For this review, take the finished solid that the model builds, in its own axes (mm). Give positions to 0.01 mm unless a question says otherwise; leave off trailing zeros. Order: outer loops, then holes, each group sorted by start corner. A loop starts at its lowest first (then second) coordinate and runs counter-clockwise, first axis right, second up. Notation, with made-up numbers: M 1,11.25 L 11,11.25 A23 ccw 11,50.25 Z; hole C 70,-22 d9. An arc over 180 degrees is marked long. Answer as CSV lines item,"result". Start each with the question number.
1. Clearance check with flat-ended pins moving along their axes: P1, Ø1.5, axis at y = -1, z = -24, coming from the -X side; P2, Ø1.5, axis at y = -1.5, z = -10, coming from the +X side. State where each tip first meets the part, or that it passes through.
2. For line 1 along X through (y, z) = (-0.2, -17); line 2 along Z through (x, y) = (39.5, -1.1); line 3 along Z through (x, y) = (-22.5, -0.4), list the stretches that pass through material, from the lowest coordinate up.
3. We need section B-B, the plane z = -11. Give the boundary of the cut face in (x, y).
4. We need section C-C, the plane y = -2.55. State how many separate pieces and enclosed holes the cut face has, and give its area (3 significant figures).
5. We need section D-D, the plane z = -28. Give the boundary of the cut face in (x, y).
6. We need section A-A, the plane x = -39. Give the boundary of the cut face in (y, z).
from build123d import *

# Parameters (mm, degrees)
SKETCH1_W          = 2.9
SKETCH1_H          = 5
SKETCH1_W_2        = 6
BASE_FLANGE1_DEPTH = 3
SKETCH25_W         = 9
SKETCH25_H         = 9.641148945
SKETCH25_W_2       = 7.205840792
CUT_EXTRUDE2_DEPTH = 10
SKETCH31_W         = 3
SKETCH31_H         = 6
CUT_EXTRUDE3_DEPTH = 10
SKETCH32_W         = 1
SKETCH32_H         = 1.138346555
SKETCH32_H_2       = 1.067484408
SKETCH32_W_2       = 1.923552289
SKETCH32_H_3       = 1
CUT_EXTRUDE4_DEPTH = 10


# Sheet-metal steps are written as plain solids
with BuildPart() as part:
    # Sketch1 → Base-Flange1 (new body)
    with BuildSketch(Plane(origin=(0, 0, 0), x_dir=(1, 0, 0), z_dir=(0, 1, 0))):
        Polygon((-80, 31.946571622), (-80, -13.053428378), (80, -13.053428378), (80, 31.946571622), (80, 41.587720567), (45, 41.587720567), (45, 31.946571622), (-45, 31.946571622), (-45, 41.587720567), (-80, 41.587720567), align=None)
        with Locations((-39.45, 10.905641405)):
            Rectangle(SKETCH1_W, SKETCH1_H, mode=Mode.SUBTRACT)
        with Locations((-22.55, 22.947848405)):
            Rectangle(SKETCH1_W, SKETCH1_H, mode=Mode.SUBTRACT)
        with Locations((-31, 22.946571622)):
            Rectangle(SKETCH1_W_2, SKETCH1_H, mode=Mode.SUBTRACT)
        with Locations((-31, 10.946571622)):
            Rectangle(SKETCH1_W_2, SKETCH1_H, mode=Mode.SUBTRACT)
        with Locations((31, 10.946571622)):
            Rectangle(SKETCH1_W_2, SKETCH1_H, mode=Mode.SUBTRACT)
        with Locations((31, 22.946571622)):
            Rectangle(SKETCH1_W_2, SKETCH1_H, mode=Mode.SUBTRACT)
        with Locations((22.55, 22.947848405)):
            Rectangle(SKETCH1_W, SKETCH1_H, mode=Mode.SUBTRACT)
        with Locations((39.45, 10.905641405)):
            Rectangle(SKETCH1_W, SKETCH1_H, mode=Mode.SUBTRACT)
    extrude(amount=-BASE_FLANGE1_DEPTH)

    # Sketch25 → Cut-Extrude2 (cut)
    with BuildSketch(Plane.XZ.offset(3)):
        Polygon((80, 13.053428378), (54, 13.053428378), (54, -31.946571622), (61.205840792, -31.946571622), (61.205840792, -41.587720567), (80, -41.587720567), align=None)
        with Locations((49.5, -36.767146095)):
            Rectangle(SKETCH25_W, SKETCH25_H)
        with Locations((57.602920396, -36.767146095)):
            Rectangle(SKETCH25_W_2, SKETCH25_H)
        with Locations((-49.5, -36.767146095)):
            Rectangle(SKETCH25_W, SKETCH25_H)
        with Locations((-57.602920396, -36.767146095)):
            Rectangle(SKETCH25_W_2, SKETCH25_H)
        Polygon((-54, -31.946571622), (-54, 13.053428378), (-80, 13.053428378), (-80, -41.587720567), (-61.205840792, -41.587720567), (-61.205840792, -31.946571622), align=None)
    extrude(amount=-CUT_EXTRUDE2_DEPTH, mode=Mode.SUBTRACT)

    # Sketch31 → Cut-Extrude3 (cut)
    with BuildSketch(Plane(origin=(0, 0, 0), x_dir=(1, 0, 0), z_dir=(0, 1, 0))):
        with Locations((52.5, 25.946571622)):
            Rectangle(SKETCH31_W, SKETCH31_H)
        with Locations((52.5, 10.946571622)):
            Rectangle(SKETCH31_W, SKETCH31_H)
        with Locations((52.5, -4.053428378)):
            Rectangle(SKETCH31_W, SKETCH31_H)
        with Locations((-52.5, 25.946571622)):
            Rectangle(SKETCH31_W, SKETCH31_H)
        with Locations((-52.5, 10.946571622)):
            Rectangle(SKETCH31_W, SKETCH31_H)
        with Locations((-52.5, -4.053428378)):
            Rectangle(SKETCH31_W, SKETCH31_H)
    extrude(amount=-CUT_EXTRUDE3_DEPTH, mode=Mode.SUBTRACT)

    # Sketch32 → Cut-Extrude4 (cut)
    with BuildSketch(Plane(origin=(0, 0, 0), x_dir=(1, 0, 0), z_dir=(0, 1, 0))):
        with Locations((-5.726537828, 16.486113061)):
            Rectangle(SKETCH32_W, SKETCH32_H)
        with Locations((-5.726537828, 9.095449689)):
            Rectangle(SKETCH32_W, SKETCH32_H_2)
        with Locations((17.1, 16.486113061)):
            Rectangle(SKETCH32_W, SKETCH32_H)
        with Locations((17.1, 9.095449689)):
            Rectangle(SKETCH32_W, SKETCH32_H_2)
        with Locations((6.311776145, 4.428231045)):
            Rectangle(SKETCH32_W_2, SKETCH32_H_3)
    extrude(amount=-CUT_EXTRUDE4_DEPTH, mode=Mode.SUBTRACT)


solid = part.part
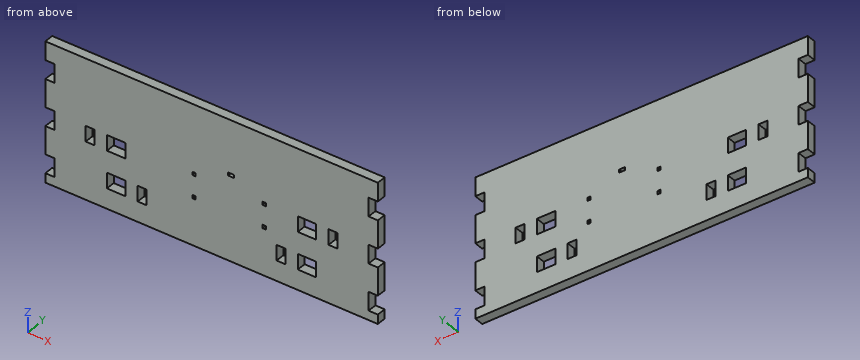
Result set:
1,P1,"x = -51"
1,P2,"x = 51"
2,line 1,"-54 to -6.23, -5.23 to 16.6, 17.6 to 54"
2,line 2,"-31.95 to -13.41, -8.41 to 13.05"
2,line 3,"-31.95 to -25.45, -20.45 to 13.05"
3,outline,"M -51,-3 L -40.9,-3 L -40.9,0 L -51,0 Z; M -38,-3 L -34,-3 L -34,0 L -38,0 Z; M -28,-3 L 28,-3 L 28,0 L -28,0 Z; M 34,-3 L 38,-3 L 38,0 L 34,0 Z; M 40.9,-3 L 51,-3 L 51,0 L 40.9,0 Z"
4,separate pieces,"1"
4,enclosed holes,"13"
4,area,"4,570 mm2"
5,outline,"M -51,-3 L 51,-3 L 51,0 L -51,0 Z"
6,outline,"M -3,-31.95 L 0,-31.95 L 0,-13.41 L -3,-13.41 Z; M -3,-8.41 L 0,-8.41 L 0,13.05 L -3,13.05 Z"
